Geometry: final body of the model. Coordinates: model frame, mm. Face numbers are marked on the shaded views. A direction names the side the tool comes from. Give positions to 0.01 mm unless a question says otherwise; leave off trailing zeros. Write each loop counter-clockwise with the first axis right and the second up, starting at its lowest first coordinate (ties: lowest second). Pieces come first, ordered by that corner, then holes.
```python
from build123d import *

# Parameters (mm, degrees)
SKETCH1_R           = 5
BOSS_EXTRUDE1_DEPTH = 7
BOSS_EXTRUDE2_START = -14
BOSS_EXTRUDE2_DEPTH = 14
SKETCH3_R           = 2.25
BOSS_EXTRUDE3_DEPTH = 3.5
CUT_EXTRUDE1_DEPTH  = 3
CIRPATTERN1_COUNT   = 6


with BuildPart() as part:
    # Sketch1 → Boss-Extrude1 (new body)
    with BuildSketch(Plane(origin=(0, 0, 0), x_dir=(1, 0, 0), z_dir=(0, 1, 0))):
        with Locations(Location((0, 0, 0), (0, 0, 270))):
            Circle(SKETCH1_R)
    extrude(amount=BOSS_EXTRUDE1_DEPTH)

    # Sketch2 → Boss-Extrude2 (add)
    with BuildSketch(Plane(origin=(0, 0, 0), x_dir=(1, 0, 0), z_dir=(0, 1, 0)).offset(BOSS_EXTRUDE2_START)):
        with BuildLine():
            Line((4, -3), (4, 3))
            ThreePointArc((4, 3), (0, 5), (-4, 3))
            Line((-4, 3), (-4, -3))
            ThreePointArc((-4, -3), (0, -5), (4, -3))
        make_face()
    extrude(amount=BOSS_EXTRUDE2_DEPTH)

    # Sketch3 → Boss-Extrude3 (add)
    with BuildSketch(Plane(origin=(0, 7, 0), x_dir=(1, 0, 0), z_dir=(0, 1, 0))):
        with Locations(Location((0, 0, 0), (0, 0, 270))):
            Circle(SKETCH3_R)
    extrude(amount=BOSS_EXTRUDE3_DEPTH)

    # Sketch4 → Cut-Extrude1 (cut)
    with BuildSketch(Plane(origin=(0, 10.5, 0), x_dir=(1, 0, 0), z_dir=(0, 1, 0))):
        Polygon((0, 1.662498522), (-5.909749561, 3.521754474), (5.909749561, 3.521754474), align=None)
    cut_extrude1 = extrude(amount=-CUT_EXTRUDE1_DEPTH, mode=Mode.SUBTRACT)

    # CirPattern1: Cut-Extrude1 ×6 about axis
    cirpattern1_axis = Axis((0, 0, 0), (0, 1, 0))
    for i in range(1, CIRPATTERN1_COUNT):
        add(cut_extrude1.rotate(cirpattern1_axis, i * 360 / CIRPATTERN1_COUNT), mode=Mode.SUBTRACT)


solid = part.part
```
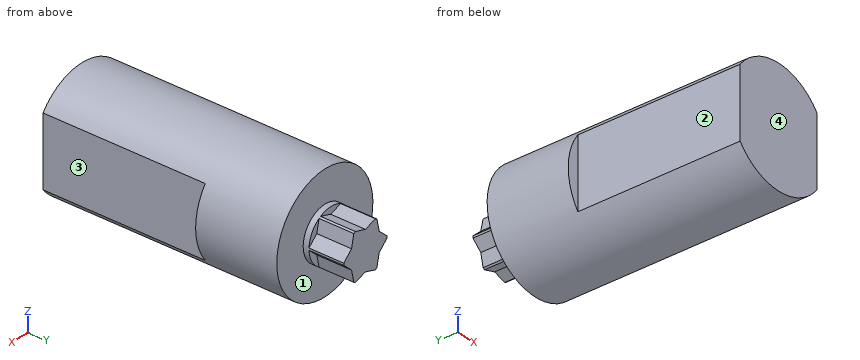
Item 1: Reachability of the marked faces 1, 2, 3 and 4 from +Z, -Z, +X, -X, +Y, -Y: full face, straight path, thin tool, end or side. Return the list, or none.
Found:
face 1: +Y
face 2: +Z, -Z, -X, -Y
face 3: +Z, -Z, +X, -Y
face 4: +Z, -Z, +X, -X, -Y
Item 2: Pin query (flat end, axial travel): pin 1 Ø6 at (x, y) = (-4, -1) entering from -Z; pin 2 Ø3 at (y, z) = (-5.5, -1) entering from -X; pin 3 Ø3 at (y, z) = (4.5, -2) entering from -X. Return the tip coordinate at first contact, or that it passes through.
Found:
pin 1: stops at z = -4.9
pin 2: stops at x = -4
pin 3: stops at x = -4.97
Item 3: Section B-B, the plane x = 0.5. Return the cut outline in (y, z).
Found:
outline: (-14, -4.97) - (7, -4.97) - (7, -2.19) - (7.5, -2.19) - (7.5, -1.82) - (10.5, -1.82) - (10.5, 1.82) - (7.5, 1.82) - (7.5, 2.19) - (7, 2.19) - (7, 4.97) - (-14, 4.97) - close
Item 4: Line query: L1, parallel to Y at x = 3.25, z = 1; L2, parallel to Z at x = -3, y = -6.75. Output: solid intervals per line, ascending.
Found:
L1: y = -14 to 7
L2: z = -4 to 4
Item 5: Section C-C, the plane z = 0.5. Return the cut outline in (x, y), plus the area to 3 significant figures.
Found:
outline: (-4.97, 0) - (-4, 0) - (-4, -14) - (4, -14) - (4, 0) - (4.97, 0) - (4.97, 7) - (2.19, 7) - (2.19, 7.5) - (1.8, 7.5) - (1.8, 10.5) - (-1.8, 10.5) - (-1.8, 7.5) - (-2.19, 7.5) - (-2.19, 7) - (-4.97, 7) - close
area: 195 mm2
Item 6: Section D-D, the plane x = -2. Return the cut outline in (y, z), plus the area to 3 significant figures.
Found:
outline: (-14, -4.58) - (7, -4.58) - (7, -1.03) - (7.5, -1.03) - (7.5, -0.32) - (10.5, -0.32) - (10.5, 0.32) - (7.5, 0.32) - (7.5, 1.03) - (7, 1.03) - (7, 4.58) - (-14, 4.58) - close
area: 195 mm2
Item 7: Section A-A, the plane y = 8.5. Return the cut outline in (x, z).
Found:
outline: (-2.25, -0.09) - (-1.44, -0.83) - (-1.2, -1.9) arc R2.25 ccw to (-1.05, -1.99) - (0, -1.66) - (1.05, -1.99) arc R2.25 ccw to (1.2, -1.9) - (1.44, -0.83) - (2.25, -0.09) arc R2.25 ccw to (2.25, 0.09) - (1.44, 0.83) - (1.2, 1.9) arc R2.25 ccw to (1.05, 1.99) - (0, 1.66) - (-1.05, 1.99) arc R2.25 ccw to (-1.2, 1.9) - (-1.44, 0.83) - (-2.25, 0.09) arc R2.25 ccw to start
